Read the model definition and answer for the solid it produces. Units are mm, in the model's axes. A direction names the side the tool comes from. Coordinates: 2 decimals unless noted, no trailing zeros. Loops run counter-clockwise (first coordinate to the right, second up) from the corner with the lowest first, then second, coordinate; pieces in that order, holes last. Notation, with made-up numbers: (62, 45) - (98, 45) arc R14 cw to (98, 50) - close; hole circle Ø9 at (-25.5, 27.5). An arc over 180 degrees is marked (long way). Use one line per item in the form item = value.
from build123d import *

# Parameters (mm, degrees)
SKETCH1_R           = 59.8
SKETCH1_R_2         = 54.8
BOSS_EXTRUDE1_DEPTH = 55
BOSS_EXTRUDE2_START = 12
SKETCH2_R           = 59.8
SKETCH2_R_2         = 15
SKETCH2_R_3         = 5.55625
BOSS_EXTRUDE2_DEPTH = 12


with BuildPart() as part:
    # Sketch1 → Boss-Extrude1 (new body)
    with BuildSketch(Plane.XY):
        Circle(SKETCH1_R)
        Circle(SKETCH1_R_2, mode=Mode.SUBTRACT)
    extrude(amount=BOSS_EXTRUDE1_DEPTH)

    # Sketch2 → Boss-Extrude2 (add)
    with BuildSketch(Plane(origin=(0, 0, 0), x_dir=(-1, 0, 0), z_dir=(0, 0, -1)).offset(BOSS_EXTRUDE2_START)):
        Circle(SKETCH2_R)
        Circle(SKETCH2_R_2, mode=Mode.SUBTRACT)
        with Locations((34.9, 0)):
            Circle(SKETCH2_R_3, mode=Mode.SUBTRACT)
    extrude(amount=-BOSS_EXTRUDE2_DEPTH)


solid = part.part
Item 1: Find the intervals of material crossed by L1, parallel to Z at x = -22.5, y = 22.5; L2, parallel to Y at x = 42.5, z = 25; L3, parallel to Y at x = 0, z = 12, in increasing order.
Results below:
L1 = -12 to 0
L2 = -42.07 to -34.59, 34.59 to 42.07
L3 = -59.8 to -54.8, 54.8 to 59.8
Item 2: The part is cut by section C-C on z = 31. Give the vertices of the cut face in (x, y).
Results below:
outline = circle Ø119.6 at (0, 0); hole circle Ø109.6 at (0, 0)
Item 3: The part is cut by section D-D on x = 38. Give the vertices of the cut face in (y, z), plus the area to 3 significant figures.
Results below:
outline = (-46.17, -12) - (46.17, -12) - (46.17, 55) - (39.48, 55) - (39.48, 0) - (-39.48, 0) - (-39.48, 55) - (-46.17, 55) - close
area = 1,840 mm²
Item 4: Which of the six approach directions +Z, -Z, +X, -X, +Y, -Y give full straight-line access (tool end or side, diameter ignored) to faces 4 (the cylindrical face through (14.985, 0.66, -6.084)), 5 (the flat face through (-11, -11, 0))?
Results below:
face_4 = +Z, -Z
face_5 = +Z
Item 5: The part is cut by section A-A on x = 0. Give the vertices of the cut face in (y, z).
Results below:
outline = (-59.8, -12) - (-15, -12) - (-15, 0) - (-54.8, 0) - (-54.8, 55) - (-59.8, 55) - close; (15, -12) - (59.8, -12) - (59.8, 55) - (54.8, 55) - (54.8, 0) - (15, 0) - close
Item 6: Each of these flat-tipped pins is pushed along its axis until it touches: P1, Ø10, axis at y = 1.5, z = 36, coming from the -X side; P2, Ø12, axis at y = 18, z = 0.5, coming from the +X side; P3, Ø6, axis at x = 36.5, z = 44, coming from the -Y side; P4, Ø10, axis at x = 20.5, y = 26, coming from the +Z side. Where does it stop, or does it pass through?
Results below:
P1 = -59.8
P2 = 58.58
P3 = -49.54
P4 = 0
Item 7: For a pull along Y with two mould halves and no side action, classify faces 1 (the flat face through (-12, -12, -12)), 2 (the cylindrical face through (-40.39, 37.036, 27.115)), 3 (the cylindrical face through (-29.35, 0.24, -6.08)) as +Y half, -Y half, draft (parallel to the pull), parting line (faces both ways), or undercut.
Results below:
face_1 = draft
face_2 = undercut
face_3 = undercut
Item 8: The part is cut by section B-B on y = 0. Give the vertices of the cut face in (x, z).
Results below:
outline = (-59.8, -12) - (-40.46, -12) - (-40.46, 0) - (-54.8, 0) - (-54.8, 55) - (-59.8, 55) - close; (-29.34, -12) - (-15, -12) - (-15, 0) - (-29.34, 0) - close; (15, -12) - (59.8, -12) - (59.8, 55) - (54.8, 55) - (54.8, 0) - (15, 0) - close
